For this review, use the dimensioned drawing (mm, ordinates from the lowest corner) and the shaded views. Give positions to 0.01 mm unless a question says otherwise; leave off trailing zeros. Order: outer loops, then holes, each group sorted by start corner. A loop starts at its lowest first (then second) coordinate and runs counter-clockwise, first axis right, second up. Notation, with made-up numbers: M -16.75,65 L 37.25,65 A30 cw 37.25,96 Z; hole C 43.5,0 d10. An arc over 180 degrees is marked long. Answer as CSV lines item,"result". Start each with the question number.
1. We need section A-A, the plane y = 33.15. Give the boundary of the cut face in (x, z), and give its area (3 significant figures).
2. For line 1 along Y through (x, z) = (99.1, 3.95); line 2 along X through (y, z) = (6.5, 2.3); line 3 along Y through (x, z) = (22.75, 1.4), list the stretches that pass through material, from the lowest coordinate up.
3. We need section B-B, the plane x = 78.5. Give the boundary of the cut face in (y, z), and give its area (3 significant figures).
4. We need section D-D, the plane x = 57.9. Give the boundary of the cut face in (y, z).
5. We need section C-C, the plane z = 1.2. Give the boundary of the cut face in (x, y), and give its area (3 significant figures).
6. Clearance check with a flat-ended pin moving along its axis: P1, Ø12.5, axis at x = 134.25, y = 20, coming from the -Z side. State where the tip first meets the part, or that it passes through.
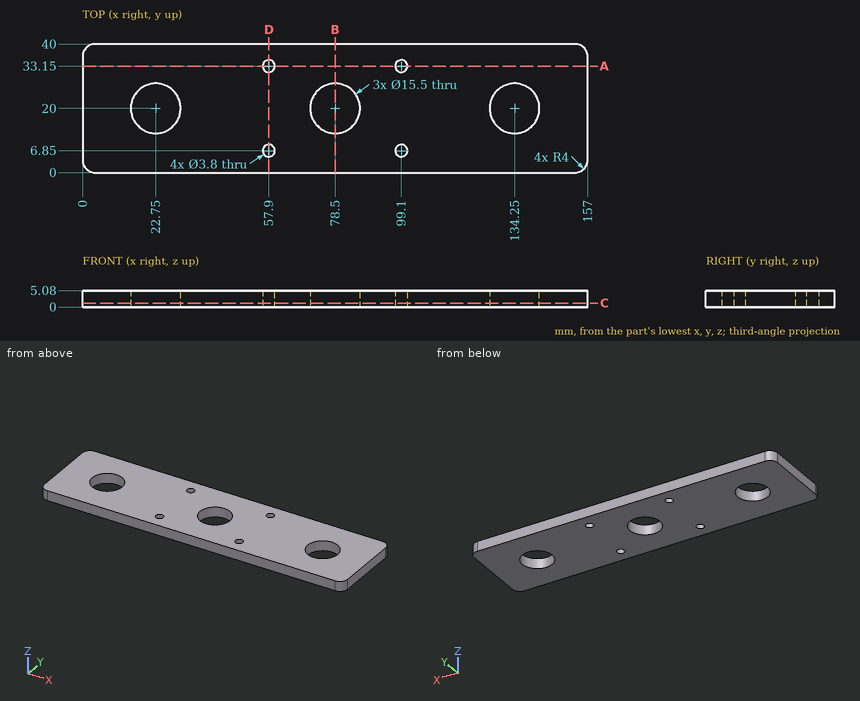
Result set:
1,outline,"M 0,0 L 56,0 L 56,5.08 L 0,5.08 Z; M 59.8,0 L 97.2,0 L 97.2,5.08 L 59.8,5.08 Z; M 101,0 L 157,0 L 157,5.08 L 101,5.08 Z"
1,area,"759 mm2"
2,line 1,"0 to 4.95, 8.75 to 31.25, 35.05 to 40"
2,line 2,"0 to 56.03, 59.77 to 97.23, 100.97 to 157"
2,line 3,"0 to 12.25, 27.75 to 40"
3,outline,"M 0,0 L 12.25,0 L 12.25,5.08 L 0,5.08 Z; M 27.75,0 L 40,0 L 40,5.08 L 27.75,5.08 Z"
3,area,"124 mm2"
4,outline,"M 0,0 L 4.95,0 L 4.95,5.08 L 0,5.08 Z; M 8.75,0 L 31.25,0 L 31.25,5.08 L 8.75,5.08 Z; M 35.05,0 L 40,0 L 40,5.08 L 35.05,5.08 Z"
5,outline,"M 0,4 A4 ccw 4,0 L 153,0 A4 ccw 157,4 L 157,36 A4 ccw 153,40 L 4,40 A4 ccw 0,36 Z; hole C 22.75,20 d15.5; hole C 57.9,6.85 d3.8; hole C 57.9,33.15 d3.8; hole C 78.5,20 d15.5; hole C 99.1,6.85 d3.8; hole C 99.1,33.15 d3.8; hole C 134.25,20 d15.5"
5,area,"5,650 mm2"
6,P1,"through"
